For this review, take the finished solid that the model builds, in its own axes (mm). A direction names the side the tool comes from. Round coordinates to 2 decimals unless told otherwise and drop trailing zeros. Order: outer loops, then holes, each group sorted by start corner. A loop starts at its lowest first (then second) coordinate and runs counter-clockwise, first axis right, second up. Notation, with made-up numbers: M 43.5,35.5 L 66.5,35.5 A7 ccw 66.5,40.5 Z; hole C 58,64 d9. An arc over 180 degrees is marked long. Answer as a JSON object with one key per item and string values.
from build123d import *

# Parameters (mm, degrees)
F1_DEPTH = 60
F2_R     = 4.5
F3_DEPTH = 25
F4_R     = 5.5
F5_DEPTH = 25
F6_R     = 5
F7_DEPTH = 25


with BuildPart() as f1:
    # F0 (on Top) → F1 (new body)
    with BuildSketch(Plane.XY):
        with BuildLine():
            Line((-30.144934, 23.315217), (29.855066, 23.315217))
            Line((29.855066, 23.315217), (29.855066, 28.315217))
            Line((29.855066, 28.315217), (-30.144934, 28.315217))
            ThreePointArc((-30.144934, 28.315217), (-37.216002, 25.386285), (-40.144934, 18.315217))
            Line((-40.144934, 18.315217), (-40.144934, -11.684783))
            ThreePointArc((-40.144934, -11.684783), (-41.6094, -15.220316), (-45.144934, -16.684783))
            Line((-45.144934, -16.684783), (-80.144934, -16.684783))
            Line((-80.144934, -16.684783), (-80.144934, -21.684783))
            Line((-80.144934, -21.684783), (-45.144934, -21.684783))
            ThreePointArc((-45.144934, -21.684783), (-38.073867, -18.75585), (-35.144934, -11.684783))
            Line((-35.144934, -11.684783), (-35.144934, 18.315217))
            ThreePointArc((-35.144934, 18.315217), (-33.680468, 21.850751), (-30.144934, 23.315217))
        make_face()
    extrude(amount=F1_DEPTH)

    # F2 (on face) → F3 (cut)
    with BuildSketch(Plane.XZ.offset(21.684783)):
        with Locations((-60.144934, 50)):
            Circle(F2_R)
        with Locations((-60.144934, 10)):
            Circle(F2_R)
    extrude(amount=-F3_DEPTH, mode=Mode.SUBTRACT)

    # F4 (on face) → F5 (cut)
    with BuildSketch(Plane.XZ.offset(-23.315217)):
        with Locations((14.855066, 30)):
            Circle(F4_R)
        with Locations((-15.144934, 30)):
            Circle(F4_R)
    extrude(amount=-F5_DEPTH, mode=Mode.SUBTRACT)

    # F6 (on face) → F7 (cut)
    with BuildSketch(Plane(origin=(-40.144934, 0, 0), x_dir=(0, -1, 0), z_dir=(-1, 0, 0))):
        with Locations((1.684783, 30)):
            Circle(F6_R)
    extrude(amount=-F7_DEPTH, mode=Mode.SUBTRACT)


solid = f1.part
1) Add section D-D on z = 38. State the section outline as (x, y) points, and give its area (3 significant figures).
Geometry check:
{"outline": "M -80.14,-21.68 L -45.14,-21.68 A10 ccw -35.14,-11.68 L -35.14,18.32 A5 cw -30.14,23.32 L 29.86,23.32 L 29.86,28.32 L -30.14,28.32 A10 ccw -40.14,18.32 L -40.14,-11.68 A5 cw -45.14,-16.68 L -80.14,-16.68 Z", "area": "743 mm²"}
2) Insertion check: P1, Ø1, axis at y = 2, z = 29.5, coming from the +X side; P2, Ø11.5, axis at y = -1.68, z = 30, coming from the +X side; P3, Ø6, axis at x = -3, z = 26.5, coming from the -Y side; P4, Ø17.5, axis at x = 14.86, z = 30, coming from the +Y side. Each pin has a flat end and moves straight along its axis. Give the tip position at first contact, or say it passes through.
Geometry check:
{"P1": "passes through", "P2": "stops at x = -35.14", "P3": "stops at y = 23.32", "P4": "stops at y = 28.32"}
3) Add section A-A on z = 30. State the section outline as (x, y) points, and give its area (3 significant figures).
Geometry check:
{"outline": "M -80.14,-21.68 L -45.14,-21.68 A10 ccw -35.14,-11.68 L -35.14,-6.68 L -40.14,-6.68 L -40.14,-11.68 A5 cw -45.14,-16.68 L -80.14,-16.68 Z; M -40.14,3.32 L -35.14,3.32 L -35.14,18.32 A5 cw -30.14,23.32 L -20.64,23.32 L -20.64,28.32 L -30.14,28.32 A10 ccw -40.14,18.32 Z; M -9.64,23.32 L 9.36,23.32 L 9.36,28.32 L -9.64,28.32 Z; M 20.36,23.32 L 29.86,23.32 L 29.86,28.32 L 20.36,28.32 Z", "area": "583 mm²"}
4) Mouldability with a two-part tool opening along X and no side actions: class faces 1 (the cylindrical face through (-41.57, -15.18, 29.58)), 2 (the cylindrical face through (-15.861, 25.78, 35.453)), 3 (the flat face through (-63, -21.685, 30)) as +X half, -X half, draft (parallel to the pull), parting line (faces both ways), or undercut.
Geometry check:
{"face 1": "-X half", "face 2": "undercut", "face 3": "draft"}
5) Machinability: for faces 4 (the flat face through (-80.145, -19, 30)), 5 (the flat face through (-35.145, 6, 30)), 6 (the flat face through (-40.145, 4, 30)), which of the approach directions +Z, -Z, +X, -X, +Y, -Y give a long, thin tool a straight path to every point of the face, cutting with its end or side? Answer none if there is none.
Geometry check:
{"face 4": "+Z, -Z, -X, +Y, -Y", "face 5": "+Z, -Z, +X, -Y", "face 6": "+Z, -Z, -X, +Y"}
6) Add section B-B on z = 50. State the section outline as (x, y) points, and give its area (3 significant figures).
Geometry check:
{"outline": "M -80.14,-21.68 L -64.64,-21.68 L -64.64,-16.68 L -80.14,-16.68 Z; M -55.64,-21.68 L -45.14,-21.68 A10 ccw -35.14,-11.68 L -35.14,18.32 A5 cw -30.14,23.32 L 29.86,23.32 L 29.86,28.32 L -30.14,28.32 A10 ccw -40.14,18.32 L -40.14,-11.68 A5 cw -45.14,-16.68 L -55.64,-16.68 Z", "area": "698 mm²"}
7) Add section C-C on y = -2. State the section outline as (x, z) points.
Geometry check:
{"outline": "M -40.14,0 L -35.14,0 L -35.14,25.01 L -40.14,25.01 Z; M -40.14,34.99 L -35.14,34.99 L -35.14,60 L -40.14,60 Z"}
8) For L1, parallel to X at y = 3, z = 13; L2, parallel to Y at x = -45, z = 54; L3, parallel to Y at x = -19, z = 23, list the stretches that pass through material, from the lowest coordinate up.
Geometry check:
{"L1": "x = -40.14 to -35.14", "L2": "y = -21.68 to -16.68", "L3": "y = 23.32 to 28.32"}
